Read the model definition and answer for the solid it produces. Units are mm, in the model's axes. A direction names the side the tool comes from. Give positions to 0.01 mm unless a question says otherwise; leave off trailing zeros. Order: outer loops, then holes, each group sorted by start corner. A loop starts at its lowest first (then second) coordinate and runs counter-clockwise, first axis right, second up. Notation, with made-up numbers: (81.5, -23.5) -> (87.5, -23.5) arc R23 cw to (87.5, -9.5) -> close; hole circle Ø1 at (-22, 32). An arc over 180 degrees is marked (long way). Answer as CSV lines item,"result". Start each with the question number.
1) Straight lines are drawn through the part: L1, parallel to X at y = -18.25, z = 25.4; L2, parallel to X at y = -14.25, z = 8.5; L3, parallel to Z at x = 27, y = -8.75. For each, find the intervals that lie inside material, in ascending order. Write a range as from..to.
2) Find section D-D (y = -16). Determine the outline of the cut face in (x, z).
3) Find section B-B (x = 2). Determine the outline of the cut face in (y, z).
4) Find section C-C (y = -7.75). Determine the outline of the cut face in (x, z), and give its area (3 significant figures).
5) The mould has two halves that part along Z. Classify faces 1 (the face through (-12, -13, 0)), 2 (the face through (-6.35, -12.56, 6.44)), 3 (the face through (-24.35, -12.88, 31.6)): +Z half, -Z half, draft (parallel to the pull), parting line (faces both ways), or undercut.
6) Find section A-A (z = 5). Determine the outline of the cut face in (x, y).
7) For faces 4 (the face through (-0.328, -13, 6)), 5 (the face through (-13.028, -13, 19)), 6 (the face through (-38.428, -13, 13)), determine the directions among +Z, -Z, +X, -X, +Y, -Y from which every point of the face is accessible in a straight line to the end or side of a thin tool.
8) Flat-ended cylindrical pins translate along their axes: pin 1 Ø12 at (y, z) = (-3, 13) entering from +X; pin 2 Ø6.5 at (y, z) = (-15.5, 20) entering from +X; pin 3 Ø6 at (y, z) = (-11.5, 29.5) entering from -X. Find the tip coordinate at first contact, or state that the pin passes through.
```python
from build123d import *

# Parameters (mm, degrees)
F1_DEPTH = 25.4
F3_DEPTH = 25.401
F5_DEPTH = 12.701


with BuildPart() as f1:
    # F0 (on Front) → F1 (new body)
    with BuildSketch(Plane.XZ):
        Polygon((-38.4284471544, 38.1), (-38.4284471544, 0), (31.4215528456, 0), (31.4215528456, 12.7), (-13.0284471544, 12.7), (-13.0284471544, 38.1), align=None)
    extrude(amount=F1_DEPTH)

    # F2 (on face) → F3 (cut, through all)
    with BuildSketch(Plane.XZ.offset(25.4)):
        with BuildLine():
            ThreePointArc((-38.4284471544, 25.4), (-34.7087032754, 34.3802561211), (-25.7284471544, 38.1))
            Line((-25.7284471544, 38.1), (-38.4284471544, 38.1))
            Line((-38.4284471544, 38.1), (-38.4284471544, 25.4))
        make_face()
        with BuildLine():
            ThreePointArc((-25.7284471544, 38.1), (-16.7481910333, 34.3802561211), (-13.0284471544, 25.4))
            Line((-13.0284471544, 25.4), (-13.0284471544, 38.1))
            Line((-13.0284471544, 38.1), (-25.7284471544, 38.1))
        make_face()
        with BuildLine():
            Line((-32.0784471544, 25.4), (-19.3784471544, 25.4))
            ThreePointArc((-19.3784471544, 25.4), (-25.7284471544, 31.75), (-32.0784471544, 25.4))
        make_face()
        with BuildLine():
            ThreePointArc((-32.0784471544, 25.4), (-25.7284471544, 19.05), (-19.3784471544, 25.4))
            Line((-19.3784471544, 25.4), (-32.0784471544, 25.4))
        make_face()
    extrude(amount=-F3_DEPTH, mode=Mode.SUBTRACT)

    # F4 (on face) → F5 (cut, through all)
    with BuildSketch(Plane.XY.offset(12.7)):
        with BuildLine():
            ThreePointArc((6.35, -12.7), (4.4901280605, -8.2098719395), (0, -6.35))
            Line((0, -6.35), (0, -19.05))
            ThreePointArc((0, -19.05), (4.4901280605, -17.1901280605), (6.35, -12.7))
        make_face()
        with BuildLine():
            Line((-0.3284471544, -19.0415000171), (-0.3284471544, -6.3584999829))
            ThreePointArc((-0.3284471544, -6.3584999829), (-6.35, -12.7), (-0.3284471544, -19.0415000171))
        make_face()
        with BuildLine():
            Line((18.7215528456, -6.35), (0, -6.35))
            ThreePointArc((0, -6.35), (4.4901280605, -8.2098719395), (6.35, -12.7))
            ThreePointArc((6.35, -12.7), (4.4901280605, -17.1901280605), (0, -19.05))
            Line((0, -19.05), (18.7215528456, -19.05))
            ThreePointArc((18.7215528456, -19.05), (12.3715528456, -12.7), (18.7215528456, -6.35))
        make_face()
        with BuildLine():
            Line((18.7215528456, -19.05), (18.7215528456, -6.35))
            ThreePointArc((18.7215528456, -6.35), (12.3715528456, -12.7), (18.7215528456, -19.05))
        make_face()
        with BuildLine():
            ThreePointArc((25.0715528456, -12.7), (23.2116809062, -8.2098719395), (18.7215528456, -6.35))
            Line((18.7215528456, -6.35), (18.7215528456, -19.05))
            ThreePointArc((18.7215528456, -19.05), (23.2116809062, -17.1901280605), (25.0715528456, -12.7))
        make_face()
        with BuildLine():
            Line((31.4215528456, 0), (18.7215528456, 0))
            ThreePointArc((18.7215528456, 0), (27.7018089667, -3.7197438789), (31.4215528456, -12.7))
            Line((31.4215528456, -12.7), (31.4215528456, 0))
        make_face()
        with BuildLine():
            Line((31.4215528456, -25.4), (31.4215528456, -12.7))
            ThreePointArc((31.4215528456, -12.7), (27.7018089667, -21.6802561211), (18.7215528456, -25.4))
            Line((18.7215528456, -25.4), (31.4215528456, -25.4))
        make_face()
    extrude(amount=-F5_DEPTH, mode=Mode.SUBTRACT)


solid = f1.part
```
Findings below:
1,L1,"-38.43..-32.08, -19.38..-13.03"
1,L2,"-38.43..-6.16, -0.33..0, 24.88..31.33"
1,L3,"0..12.7"
2,outline,"(-38.43, 0) -> (-5.43, 0) -> (-5.43, 12.7) -> (-13.03, 12.7) -> (-13.03, 25.4) arc R12.7 ccw to (-38.43, 25.4) -> close; (-0.33, 0) -> (0, 0) -> (0, 12.7) -> (-0.33, 12.7) -> close; (24.15, 0) -> (30.99, 0) -> (30.99, 12.7) -> (24.15, 12.7) -> close; hole circle Ø12.7 at (-25.73, 25.4)"
3,outline,"(-25.4, 0) -> (-19.05, 0) -> (-19.05, 12.7) -> (-25.4, 12.7) -> close; (-6.35, 0) -> (0, 0) -> (0, 12.7) -> (-6.35, 12.7) -> close"
4,outline,"(-38.43, 0) -> (-3.98, 0) -> (-3.98, 12.7) -> (-13.03, 12.7) -> (-13.03, 25.4) arc R12.7 ccw to (-38.43, 25.4) -> close; (-0.33, 0) -> (0, 0) -> (0, 12.7) -> (-0.33, 12.7) -> close; (22.7, 0) -> (30.42, 0) -> (30.42, 12.7) -> (22.7, 12.7) -> close; hole circle Ø12.7 at (-25.73, 25.4)"
4,area,"989 mm²"
5,face 1,"-Z half"
5,face 2,"draft"
5,face 3,"undercut"
6,outline,"(-38.43, -25.4) -> (18.72, -25.4) arc R12.7 ccw to (18.72, 0) -> (-38.43, 0) -> close; hole (-0.33, -19.04) -> (-0.33, -6.36) arc R6.35 ccw to start; hole (0, -19.05) -> (18.72, -19.05) arc R6.35 ccw to (18.72, -6.35) -> (0, -6.35) -> close"
7,face 4,"+Z, -Z"
7,face 5,"+Z, +X, +Y, -Y"
7,face 6,"+Z, -Z, -X, +Y, -Y"
8,pin 1,"x = 30.87"
8,pin 2,"x = -13.03"
8,pin 3,"x = -38.38"
